The figure shows three views and two pictorial views of one solid part (mm, origin at its lowest corner). Answer the questions. Coordinates: 2 decimals unless noted, no trailing zeros. Order: outer loops, then holes, each group sorted by start corner. A loop starts at its lowest first (then second) coordinate and runs counter-clockwise, first axis right, second up. Notation, with made-up numbers: (62.25, 8) -> (90.25, 8) arc R30 cw to (90.25, 32) -> close; hole circle Ø5 at (15.5, -14.75). An arc over 180 degrees is marked (long way). Write item = value, one per line.
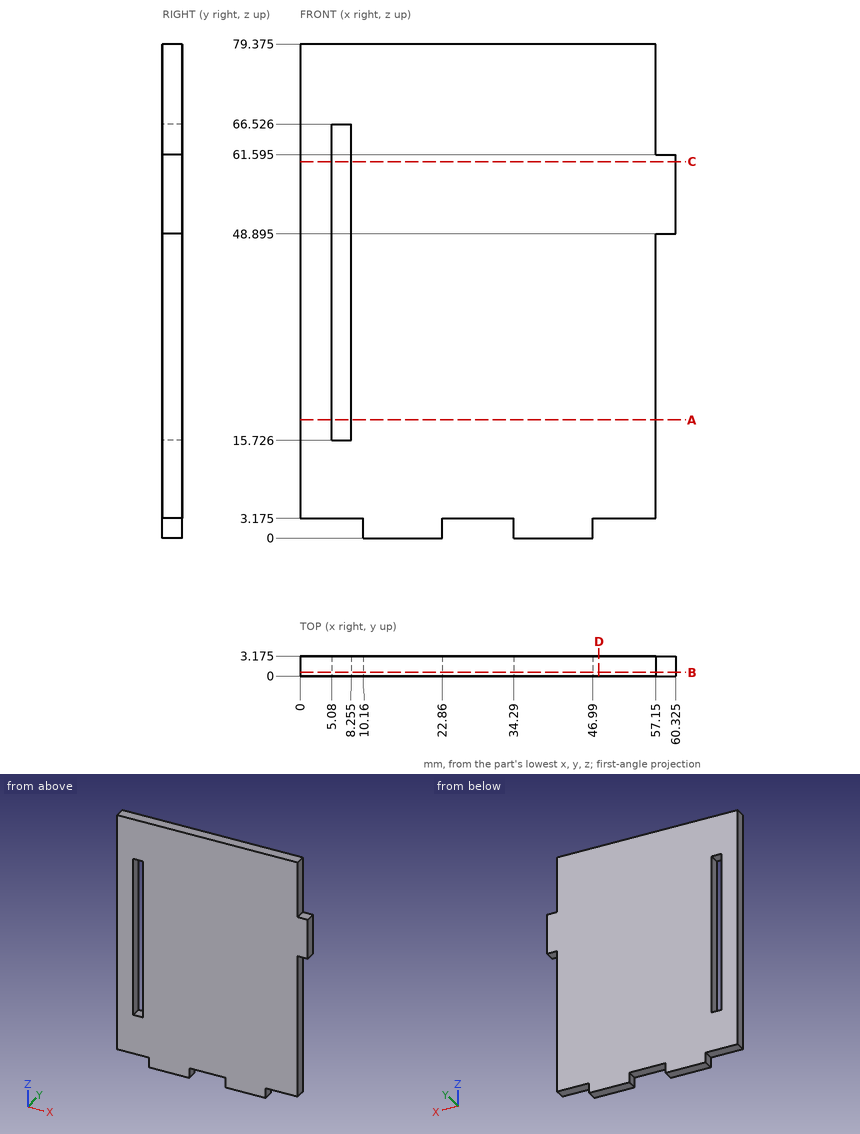
Q1. Each of these flat-tipped pins is pushed along its axis until it touches: pin 1 Ø1.6 at (y, z) = (1.5, 1) entering from +X; pin 2 Ø1 at (x, z) = (30, 13) entering from -Y; pin 3 Ø1 at (y, z) = (1.5, 71) entering from +X; pin 4 Ø1.6 at (x, y) = (53.5, 2) entering from -Z (3 decimals). Where does it stop, or does it pass through?
The answers:
pin_1 = 46.99
pin_2 = 0
pin_3 = 57.15
pin_4 = 3.175
Q2. Find the intervals of material crossed by line 1 along X through (y, z) = (0.4, 63) (3 decimals); line 2 along Z through (x, y) = (6, 1.65) (3 decimals); line 3 along X through (y, z) = (0.6, 60) (3 decimals), in increasing order.
The answers:
line_1 = 0 to 5.08, 8.255 to 57.15
line_2 = 3.175 to 15.726, 66.526 to 79.375
line_3 = 0 to 5.08, 8.255 to 60.325
Q3. Section B-B, the plane y = 0.6 is taken. Give the vertices of the cut face in (x, z) (3 decimals), plus the area to 3 significant figures.
The answers:
outline = (0, 3.175) -> (10.16, 3.175) -> (10.16, 0) -> (22.86, 0) -> (22.86, 3.175) -> (34.29, 3.175) -> (34.29, 0) -> (46.99, 0) -> (46.99, 3.175) -> (57.15, 3.175) -> (57.15, 48.895) -> (60.325, 48.895) -> (60.325, 61.595) -> (57.15, 61.595) -> (57.15, 79.375) -> (0, 79.375) -> close; hole (5.08, 15.726) -> (8.255, 15.726) -> (8.255, 66.526) -> (5.08, 66.526) -> close
area = 4,310 mm2
Q4. Section D-D, the plane x = 48 is taken. Give the vertices of the cut face in (y, z) (3 decimals).
The answers:
outline = (0, 3.175) -> (3.175, 3.175) -> (3.175, 79.375) -> (0, 79.375) -> close
Q5. Section C-C, the plane z = 60.5 is taken. Give the vertices of the cut face in (x, y) (3 decimals).
The answers:
outline = (0, 0) -> (5.08, 0) -> (5.08, 3.175) -> (0, 3.175) -> close; (8.255, 0) -> (60.325, 0) -> (60.325, 3.175) -> (8.255, 3.175) -> close
Q6. Section A-A, the plane z = 19 is taken. Give the vertices of the cut face in (x, y) (3 decimals).
The answers:
outline = (0, 0) -> (5.08, 0) -> (5.08, 3.175) -> (0, 3.175) -> close; (8.255, 0) -> (57.15, 0) -> (57.15, 3.175) -> (8.255, 3.175) -> close
